Answer from the drawing. Dimensions are ordinates in mm from the lowest x, y and z of the part. Give positions to 0.01 mm unless a question says otherwise; leave off trailing zeros. Loops run counter-clockwise (first coordinate to the right, second up) from the corner with the lowest first, then second, coordinate; pieces in that order, holes last. Notation, with made-up numbers: (52.5, 69) - (97.5, 69) arc R30 ccw to (97.5, 103) - close; hole circle Ø1 at (67, 57). An arc over 180 degrees is marked (long way). Put each result on its own line as item: value. Start each with the question number.
1. A cutting plane is placed at C-C, the plane x = 43. Determine the outline of the cut face in (y, z).
2. For a pull along X with two mould halves and no side action, classify the marked faces 1, 2, 3 and 4 as released by +X, released by -X, zero draft, split by the parting line, or undercut.
3. Given pin 1 Ø4 at (x, z) = (7, 39) entering from +Y, flat-ended and moving along its own axis, determine where the tip first touches the part or whether it passes through.
4. Consider L1, parallel to Z at x = 7, y = 10; L2, parallel to X at y = 22, z = 38.5; L3, parallel to Z at x = 6, y = 26. Determine where each line is inside the solid, lowest interval first. Write a range as from..to.
5. A cutting plane is placed at A-A, the plane z = 5. Determine the outline of the cut face in (x, y), plus the area to 3 significant figures.
6. A cutting plane is placed at B-B, the plane y = 13. Determine the outline of the cut face in (x, z), plus the area to 3 significant figures.
7. A cutting plane is placed at D-D, the plane z = 31. Determine the outline of the cut face in (x, y), plus the area to 3 significant figures.
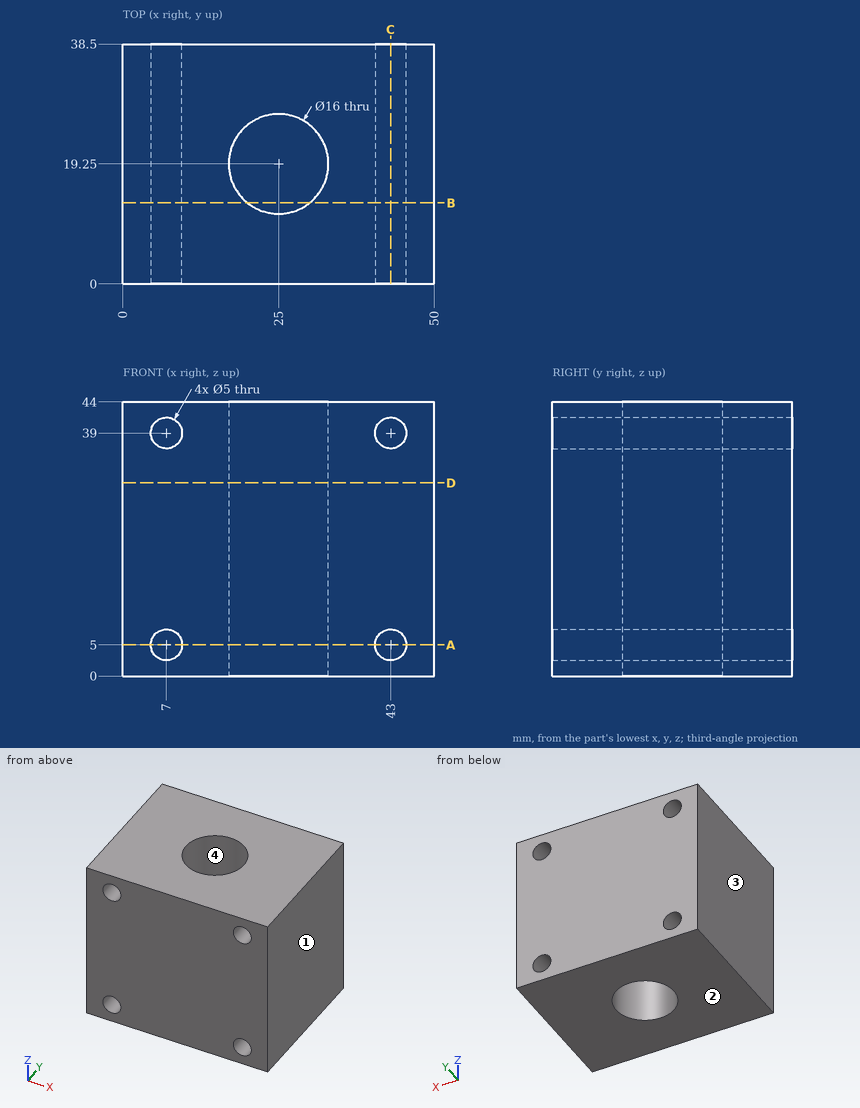
Return value:
1. outline: (0, 0) - (38.5, 0) - (38.5, 2.5) - (0, 2.5) - close; (0, 7.5) - (38.5, 7.5) - (38.5, 36.5) - (0, 36.5) - close; (0, 41.5) - (38.5, 41.5) - (38.5, 44) - (0, 44) - close
2. face 1: released by +X
2. face 2: zero draft
2. face 3: released by -X
2. face 4: undercut
3. pin 1: passes through
4. L1: z = 0..2.5, 7.5..36.5, 41.5..44
4. L2: x = 0..4.55, 9.45..17.49, 32.51..40.55, 45.45..50
4. L3: z = 0..2.71, 7.29..36.71, 41.29..44
5. outline: (0, 0) - (4.5, 0) - (4.5, 38.5) - (0, 38.5) - close; (9.5, 0) - (40.5, 0) - (40.5, 38.5) - (9.5, 38.5) - close; (45.5, 0) - (50, 0) - (50, 38.5) - (45.5, 38.5) - close; hole circle Ø16 at (25, 19.25)
5. area: 1,340 mm2
6. outline: (0, 0) - (20.01, 0) - (20.01, 44) - (0, 44) - close; (29.99, 0) - (50, 0) - (50, 44) - (29.99, 44) - close; hole circle Ø5 at (7, 5); hole circle Ø5 at (7, 39); hole circle Ø5 at (43, 5); hole circle Ø5 at (43, 39)
6. area: 1,680 mm2
7. outline: (0, 0) - (50, 0) - (50, 38.5) - (0, 38.5) - close; hole circle Ø16 at (25, 19.25)
7. area: 1,720 mm2
